Source: CAD feature listing. Evaluate the final solid. Frame: model axes, mm. Face numbers are marked on the shaded views. A direction names the side the tool comes from. Give positions to 0.01 mm unless a question says otherwise; leave off trailing zeros. Write each loop counter-clockwise with the first axis right and the second up, starting at its lowest first coordinate (ties: lowest second). Pieces come first, ordered by that corner, then holes. Notation, with made-up numbers: (52.5, -24.75) - (101.5, -24.75) arc R8 cw to (101.5, -16.75) - close; hole circle Ø5 at (-24, 16.5). An arc over 180 degrees is marked (long way). Answer as a JSON object with one key per item and string values. Group by question number.
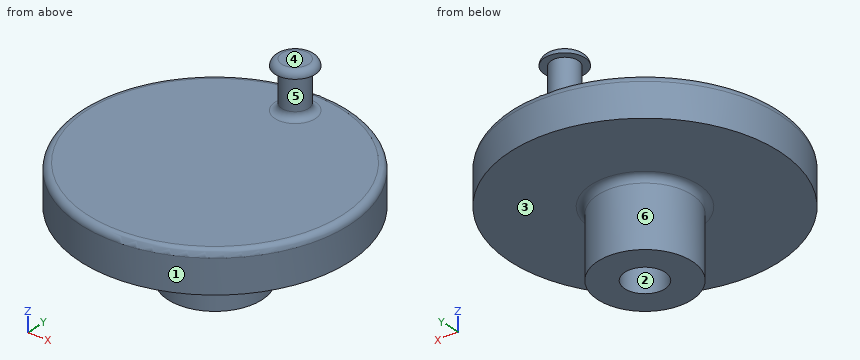
from build123d import *

# Parameters (mm, degrees)
SKETCH1_R           = 20
BOSS_EXTRUDE1_DEPTH = 6
SKETCH2_R           = 7
SKETCH2_R_2         = 3
BOSS_EXTRUDE2_DEPTH = 10
SKETCH3_R           = 2
BOSS_EXTRUDE3_DEPTH = 7
SKETCH4_R           = 3
BOSS_EXTRUDE4_DEPTH = 1
FILLET1_R           = 1


with BuildPart() as part:
    # Sketch1 → Boss-Extrude1 (new body)
    with BuildSketch(Plane.XY):
        Circle(SKETCH1_R)
    extrude(amount=BOSS_EXTRUDE1_DEPTH)

    # Sketch2 → Boss-Extrude2 (add)
    with BuildSketch(Plane(origin=(0, 0, 0), x_dir=(-1, 0, 0), z_dir=(0, 0, -1))):
        with Locations(Location((0, 0, 0), (0, 0, 180))):
            Circle(SKETCH2_R)
        Circle(SKETCH2_R_2, mode=Mode.SUBTRACT)
    extrude(amount=BOSS_EXTRUDE2_DEPTH)

    # Sketch3 → Boss-Extrude3 (add)
    with BuildSketch(Plane.XY.offset(6)):
        with Locations((0, 15)):
            Circle(SKETCH3_R)
    extrude(amount=BOSS_EXTRUDE3_DEPTH)

    # Sketch4 → Boss-Extrude4 (add)
    with BuildSketch(Plane.XY.offset(13)):
        with Locations((0, 15)):
            Circle(SKETCH4_R)
    extrude(amount=-BOSS_EXTRUDE4_DEPTH)

    # Fillet1
    fillet1_edges = [part.edges().sort_by_distance(p)[0] for p in [
        (-2, 15, 6),
        (-3, 15, 13),
        (-20, 0, 6),
        (-7, 0, 0),
    ]]
    fillet(fillet1_edges, radius=FILLET1_R - 0.0001)  # a hair under: the kernel refuses the full size


solid = part.part
Q1. Section C-C on z = 2. Return the cut outline in (x, y).
Q2. Section A-A on y = 0. Return the cut outline in (x, z).
Q3. Ray query, probe 1 along Y at (x, z) = (0, -3.75); probe 2 along Z at (x, y) = (-8, 0); probe 3 along X at (y, z) = (-2, -4.75). Return the intervals inside material, ascending. Write a range as [from, to].
Q4. First-contact query: pin 1 Ø5 at (x, y) = (1, 0.5) entering from -Z; pin 2 Ø8 at (x, z) = (11.5, 2) entering from -Y; pin 3 Ø5.5 at (x, y) = (0, 0) entering from -Z; pin 4 Ø4 at (y, z) = (9, 1) entering from +X (3 decimals). Flat tips, straight axial feed; report the tip coordinate or a pass-through.
Q5. Draft query along X for the marked faces 1, 2 and 3. Return one class per face: released by +X, released by -X, zero draft, split by the parting line, or undercut.
Q6. Reachability of the marked faces 4, 5 and 6 from +Z, -Z, +X, -X, +Y, -Y: full face, straight path, thin tool, end or side. Return the list, or none.
Taken from the geometry:
{
 "1": {"outline": "circle Ø40 at (0, 0)"},
 "2": {"outline": "(-20, 0) - (-8, 0) arc R1 cw to (-7, -1) - (-7, -10) - (-3, -10) - (-3, 0) - (3, 0) - (3, -10) - (7, -10) - (7, -1) arc R1 cw to (8, 0) - (20, 0) - (20, 5) arc R1 ccw to (19, 6) - (-19, 6) arc R1 ccw to (-20, 5) - close"},
 "3": {"probe 1": "y = [-7, -3], [3, 7]", "probe 2": "z = [0, 6]", "probe 3": "x = [-6.71, -2.24], [2.24, 6.71]"},
 "4": {"pin 1": "stops at z = -10", "pin 2": "stops at y = -18.54", "pin 3": "stops at z = 0", "pin 4": "stops at x = 18.735"},
 "5": {"face 1": "split by the parting line", "face 2": "undercut", "face 3": "zero draft"},
 "6": {"face 4": "+Z, +X, -X, +Y, -Y", "face 5": "none", "face 6": "-Z"}
}
